Read the model definition and answer for the solid it produces. Units are mm, in the model's axes. A direction names the side the tool comes from. Round coordinates to 2 decimals unless told otherwise and drop trailing zeros. Order: outer loops, then holes, each group sorted by start corner. A loop starts at its lowest first (then second) coordinate and runs counter-clockwise, first axis right, second up.
from build123d import *

# Parameters (mm, degrees)
SKETCH1_W           = 38.1
SKETCH1_H           = 88.9
BOSS_EXTRUDE1_DEPTH = 76.2
SKETCH2_W           = 16.51
SKETCH2_H           = 60.96
CUT_EXTRUDE1_DEPTH  = 76.2
SKETCH3_W           = 5.08
SKETCH3_H           = 46.99
SKETCH3_W_2         = 2.032
SKETCH3_W_3         = 3.81
SKETCH3_H_2         = 2.032
CUT_EXTRUDE2_DEPTH  = 89.9
SKETCH5_W           = 7.62
SKETCH5_H           = 12.7
CUT_EXTRUDE3_DEPTH  = 14.605
SKETCH6_W           = 17.78
SKETCH6_H           = 25.4
SKETCH6_W_2         = 12.7
SKETCH6_H_2         = 20.32
BOSS_EXTRUDE2_DEPTH = 12.7
FILLET2_R           = 10
SKETCH7_R           = 2.7305
CUT_EXTRUDE4_DEPTH  = 12.7


with BuildPart() as part:
    # Sketch1 → Boss-Extrude1 (new body)
    with BuildSketch(Plane(origin=(0, 0, 0), x_dir=(1, 0, 0), z_dir=(0, 1, 0))):
        with Locations((19.05, 44.45)):
            Rectangle(SKETCH1_W, SKETCH1_H)
    extrude(amount=BOSS_EXTRUDE1_DEPTH)

    # Sketch2 → Cut-Extrude1 (cut)
    with BuildSketch(Plane.XY):
        with Locations((15.875, 38.1)):
            Rectangle(SKETCH2_W, SKETCH2_H)
    extrude(amount=-CUT_EXTRUDE1_DEPTH, mode=Mode.SUBTRACT)

    # Sketch3 → Cut-Extrude2 (cut, through all)
    with BuildSketch(Plane.XY):
        with Locations((29.718, 38.1)):
            Rectangle(SKETCH3_W, SKETCH3_H)
        with Locations((33.274, 38.1)):
            Rectangle(SKETCH3_W_2, SKETCH3_H)
        with Locations((36.195, 38.1)):
            Rectangle(SKETCH3_W_3, SKETCH3_H)
        with Locations((33.274, 62.611)):
            Rectangle(SKETCH3_W_2, SKETCH3_H_2)
        with Locations((33.274, 13.589)):
            Rectangle(SKETCH3_W_2, SKETCH3_H_2)
    extrude(amount=-CUT_EXTRUDE2_DEPTH, mode=Mode.SUBTRACT)

    # Sketch5 → Cut-Extrude3 (cut)
    with BuildSketch(Plane(origin=(0, 76.2, 0), x_dir=(1, 0, 0), z_dir=(0, 1, 0))):
        with Locations((29.21, 8.89)):
            Rectangle(SKETCH5_W, SKETCH5_H)
    extrude(amount=-CUT_EXTRUDE3_DEPTH, mode=Mode.SUBTRACT)

    # Sketch6 → Boss-Extrude2 (add)
    with BuildSketch(Plane(origin=(0, 76.2, 0), x_dir=(1, 0, 0), z_dir=(0, 1, 0))):
        with Locations((29.21, 12.7)):
            Rectangle(SKETCH6_W, SKETCH6_H)
        with Locations((29.21, 12.7)):
            Rectangle(SKETCH6_W_2, SKETCH6_H_2, mode=Mode.SUBTRACT)
    extrude(amount=BOSS_EXTRUDE2_DEPTH)

    # Fillet2
    fillet2_edges = [part.edges().sort_by_distance(p)[0] for p in [
        (20.32, 76.2, -12.7),
        (0, 76.2, -44.45),
        (38.1, 0, -44.45),
        (0, 0, -44.45),
        (38.1, 76.2, -57.15),
    ]]
    fillet(fillet2_edges, radius=FILLET2_R)

    # Sketch7 → Cut-Extrude4 (cut)
    with BuildSketch(Plane(origin=(0, 0, -88.9), x_dir=(-1, 0, 0), z_dir=(0, 0, -1))):
        with Locations((-13.589, 63.5)):
            Circle(SKETCH7_R)
        with Locations((-13.589, 12.7)):
            Circle(SKETCH7_R)
    extrude(amount=-CUT_EXTRUDE4_DEPTH, mode=Mode.SUBTRACT)


solid = part.part
Q1. A cutting plane is placed at B-B, the plane y = 83. Give the vertices of the cut face in (x, z), plus the area to 3 significant figures.
Outcome:
outline: (19.79, -25.4) - (38.1, -25.4) - (38.1, 0) - (19.79, 0) - close; hole (22.86, -22.86) - (35.56, -22.86) - (35.56, -2.54) - (22.86, -2.54) - close
area: 207 mm2
Q2. A cutting plane is placed at A-A, the plane z = -54.5. Give the vertices of the cut face in (x, y) (3 decimals).
Outcome:
outline: (0, 10) arc R10 ccw to (10, 0) - (28.1, 0) arc R10 ccw to (38.1, 10) - (38.1, 14.605) - (34.29, 14.605) - (34.29, 12.573) - (32.258, 12.573) - (32.258, 14.605) - (27.178, 14.605) - (27.178, 61.595) - (32.258, 61.595) - (32.258, 63.627) - (34.29, 63.627) - (34.29, 61.595) - (38.1, 61.595) - (38.1, 66.2) arc R10 ccw to (28.1, 76.2) - (10, 76.2) arc R10 ccw to (0, 66.2) - close; hole (7.62, 7.62) - (24.13, 7.62) - (24.13, 68.58) - (7.62, 68.58) - close
Q3. Straight lines are drawn through the part: probe 1 along Y at (x, z) = (10, -72.5); probe 2 along Y at (x, z) = (27.5, -27) (3 decimals); probe 3 along X at (y, z) = (26, -46.5). For each, find the intervals that lie inside material, in ascending order.
Outcome:
probe 1: y = 0 to 7.62, 68.58 to 76.2
probe 2: y = 0 to 14.605, 61.595 to 76.2
probe 3: x = 0 to 7.62, 24.13 to 27.18
Q4. For faces 4 (the face through (32.258, 63, -52)), 5 (the face through (29, 82, -22.86)), 6 (the face through (27.178, 38, -44)), 7 (the face through (7.62, 38, -38)), determine the directions among +Z, -Z, +X, -X, +Y, -Y from which every point of the face is accessible in a straight line to the end or side of a thin tool.
Outcome:
face 4: +Z, -Z
face 5: +Y
face 6: +Z, -Z, +X
face 7: +Z
Q5. Flat-ended cylindrical pins translate along their axes: pin 1 (1.5 mm diameter, centred on x = 30.5, z = -55, fed in from +Y); pin 2 (0.6 mm diameter, centred on x = 33.5, z = -34, fed in from +Y); pin 3 (8 mm diameter, centred on x = 25.5, z = -9, fed in from +Y); pin 4 (5 mm diameter, centred on x = 16, z = -32.5, fed in from +Y). Find the tip coordinate at first contact, or state that the pin passes through.
Outcome:
pin 1: stops at y = 76.06
pin 2: stops at y = 74.8
pin 3: stops at y = 88.9
pin 4: stops at y = 76.2
Q6. For a pull along Y with two mould halves and no side action, classify faces 1 (the face through (37, 88.9, -13)), 2 (the face through (30, 61.595, -52)), 3 (the face through (35.56, 82, -13)) as released by +Y, released by -Y, zero draft, split by the parting line, or undercut.
Outcome:
face 1: released by +Y
face 2: undercut
face 3: zero draft
Q7. A cutting plane is placed at C-C, the plane z = -82. Give the vertices of the cut face in (x, y) (1 decimal).
Outcome:
outline: (0, 10) arc R10 ccw to (10, 0) - (28.1, 0) arc R10 ccw to (38.1, 10) - (38.1, 14.6) - (34.3, 14.6) - (34.3, 12.6) - (32.3, 12.6) - (32.3, 14.6) - (27.2, 14.6) - (27.2, 61.6) - (32.3, 61.6) - (32.3, 63.6) - (34.3, 63.6) - (34.3, 61.6) - (38.1, 61.6) - (38.1, 66.2) arc R10 ccw to (28.1, 76.2) - (10, 76.2) arc R10 ccw to (0, 66.2) - close; hole circle Ø5.5 at (13.6, 12.7); hole circle Ø5.5 at (13.6, 63.5)
Q8. A cutting plane is placed at D-D, the plane y = 21. Give the vertices of the cut face in (x, z), plus the area to 3 significant figures.
Outcome:
outline: (0, -88.9) - (27.18, -88.9) - (27.18, 0) - (24.13, 0) - (24.13, -76.2) - (7.62, -76.2) - (7.62, 0) - (0, 0) - close
area: 1,160 mm2
